from build123d import *

# Parameters (mm, degrees)
SKETCH1_R           = 52.5
BOSS_EXTRUDE1_DEPTH = 65


with BuildPart() as part:
    # Sketch1 → Boss-Extrude1 (new body)
    with BuildSketch(Plane(origin=(0, 0, 0), x_dir=(1, 0, 0), z_dir=(0, 1, 0))):
        with BuildLine():
            Line((0, 57), (0, 60))
            ThreePointArc((0, 60), (3.662912372, 59.888087905), (7.312160604, 59.552769098))
            Line((7.312160604, 59.552769098), (6.946552574, 56.575130644))
            ThreePointArc((6.946552574, 56.575130644), (9.407713534, 56.218279288), (11.850966377, 55.754413242))
            Line((11.850966377, 55.754413242), (12.474701449, 58.688856044))
            ThreePointArc((12.474701449, 58.688856044), (16.034302565, 57.817827193), (19.534089267, 56.731114536))
            Line((19.534089267, 56.731114536), (18.557384804, 53.894558809))
            ThreePointArc((18.557384804, 53.894558809), (20.890569923, 53.033801375), (23.183988655, 52.072091086))
            Line((23.183988655, 52.072091086), (24.404198585, 54.812727459))
            ThreePointArc((24.404198585, 54.812727459), (27.704916794, 53.220649991), (30.902284495, 51.430038042))
            Line((30.902284495, 51.430038042), (29.35717027, 48.85853614))
            ThreePointArc((29.35717027, 48.85853614), (31.460408163, 47.531491858), (33.503759381, 46.113968679))
            Line((33.503759381, 46.113968679), (35.267115138, 48.541019662))
            ThreePointArc((35.267115138, 48.541019662), (38.164693217, 46.297475003), (40.919901604, 43.881222097))
            Line((40.919901604, 43.881222097), (38.873906524, 41.687160992))
            ThreePointArc((38.873906524, 41.687160992), (40.655275602, 39.951828065), (42.359255052, 38.140444562))
            Line((42.359255052, 38.140444562), (44.588689529, 40.147836382))
            ThreePointArc((44.588689529, 40.147836382), (46.956489411, 37.350878198), (49.149122657, 34.414586181))
            Line((49.149122657, 34.414586181), (46.691666524, 32.693856872))
            ThreePointArc((46.691666524, 32.693856872), (48.073312411, 30.626077676), (49.363448016, 28.5))
            Line((49.363448016, 28.5), (51.961524227, 30))
            ThreePointArc((51.961524227, 30), (53.696061696, 26.771868787), (55.230291207, 23.443867709))
            Line((55.230291207, 23.443867709), (52.468776647, 22.271674324))
            ThreePointArc((52.468776647, 22.271674324), (53.390314787, 19.961820732), (54.210221429, 17.613968679))
            Line((54.210221429, 17.613968679), (57.063390978, 18.541019662))
            ThreePointArc((57.063390978, 18.541019662), (58.088858423, 15.022800243), (58.897631007, 11.448539723))
            Line((58.897631007, 11.448539723), (55.952749457, 10.876112736))
            ThreePointArc((55.952749457, 10.876112736), (56.373904212, 8.425136434), (56.687748036, 5.958122406))
            Line((56.687748036, 5.958122406), (59.671313722, 6.271707796))
            ThreePointArc((59.671313722, 6.271707796), (59.942893295, 2.617163242), (59.990861709, -1.047144386))
            Line((59.990861709, -1.047144386), (56.991318624, -0.994787167))
            ThreePointArc((56.991318624, -0.994787167), (56.89368351, -3.479766753), (56.687748036, -5.958122406))
            Line((56.687748036, -5.958122406), (59.671313722, -6.271707796))
            ThreePointArc((59.671313722, -6.271707796), (59.177136092, -9.902856352), (58.462203887, -13.497063261))
            Line((58.462203887, -13.497063261), (55.539093693, -12.822210098))
            ThreePointArc((55.539093693, -12.822210098), (54.926935833, -15.232587436), (54.210221429, -17.613968679))
            Line((54.210221429, -17.613968679), (57.063390978, -18.541019662))
            ThreePointArc((57.063390978, -18.541019662), (55.825054079, -21.990073603), (54.378467222, -25.357095704))
            Line((54.378467222, -25.357095704), (51.659543861, -24.089240919))
            ThreePointArc((51.659543861, -24.089240919), (50.559617491, -26.319670954), (49.363448016, -28.5))
            Line((49.363448016, -28.5), (51.961524227, -30))
            ThreePointArc((51.961524227, -30), (50.033149324, -33.116219119), (47.918130603, -36.108901389))
            Line((47.918130603, -36.108901389), (45.522224073, -34.30345632))
            ThreePointArc((45.522224073, -34.30345632), (43.982601253, -36.256458556), (42.359255052, -38.140444562))
            Line((42.359255052, -38.140444562), (44.588689529, -40.147836382))
            ThreePointArc((44.588689529, -40.147836382), (42.054555858, -42.795026949), (39.363541739, -45.282574813))
            Line((39.363541739, -45.282574813), (37.395364652, -43.018446073))
            ThreePointArc((37.395364652, -43.018446073), (35.483334288, -44.608664941), (33.503759381, -46.113968679))
            Line((33.503759381, -46.113968679), (35.267115138, -48.541019662))
            ThreePointArc((35.267115138, -48.541019662), (32.237976501, -50.603486749), (29.088577215, -52.477182428))
            Line((29.088577215, -52.477182428), (27.634148354, -49.853323307))
            ThreePointArc((27.634148354, -49.853323307), (25.433275347, -51.011258611), (23.183988655, -52.072091086))
            Line((23.183988655, -52.072091086), (24.404198585, -54.812727459))
            ThreePointArc((24.404198585, -54.812727459), (21.012442876, -56.200331355), (17.542302283, -57.378285358))
            Line((17.542302283, -57.378285358), (16.665187169, -54.50937109))
            ThreePointArc((16.665187169, -54.50937109), (14.271660231, -55.184415502), (11.850966377, -55.754413242))
            Line((11.850966377, -55.754413242), (12.474701449, -58.688856044))
            ThreePointArc((12.474701449, -58.688856044), (8.868564668, -59.340951802), (5.229344565, -59.771681886))
            Line((5.229344565, -59.771681886), (4.967877337, -56.783097791))
            ThreePointArc((4.967877337, -56.783097791), (2.48630508, -56.94574863), (0, -57))
            Line((0, -57), (0, -60))
            ThreePointArc((0, -60), (-3.662912372, -59.888087905), (-7.312160604, -59.552769098))
            Line((-7.312160604, -59.552769098), (-6.946552574, -56.575130644))
            ThreePointArc((-6.946552574, -56.575130644), (-9.407713534, -56.218279288), (-11.850966377, -55.754413242))
            Line((-11.850966377, -55.754413242), (-12.474701449, -58.688856044))
            ThreePointArc((-12.474701449, -58.688856044), (-16.034302565, -57.817827193), (-19.534089267, -56.731114536))
            Line((-19.534089267, -56.731114536), (-18.557384804, -53.894558809))
            ThreePointArc((-18.557384804, -53.894558809), (-20.890569923, -53.033801375), (-23.183988655, -52.072091086))
            Line((-23.183988655, -52.072091086), (-24.404198585, -54.812727459))
            ThreePointArc((-24.404198585, -54.812727459), (-27.704916794, -53.220649991), (-30.902284495, -51.430038042))
            Line((-30.902284495, -51.430038042), (-29.35717027, -48.85853614))
            ThreePointArc((-29.35717027, -48.85853614), (-31.460408163, -47.531491858), (-33.503759381, -46.113968679))
            Line((-33.503759381, -46.113968679), (-35.267115138, -48.541019662))
            ThreePointArc((-35.267115138, -48.541019662), (-38.164693217, -46.297475003), (-40.919901604, -43.881222097))
            Line((-40.919901604, -43.881222097), (-38.873906524, -41.687160992))
            ThreePointArc((-38.873906524, -41.687160992), (-40.655275602, -39.951828065), (-42.359255052, -38.140444562))
            Line((-42.359255052, -38.140444562), (-44.588689529, -40.147836382))
            ThreePointArc((-44.588689529, -40.147836382), (-46.956489411, -37.350878198), (-49.149122657, -34.414586181))
            Line((-49.149122657, -34.414586181), (-46.691666524, -32.693856872))
            ThreePointArc((-46.691666524, -32.693856872), (-48.073312411, -30.626077676), (-49.363448016, -28.5))
            Line((-49.363448016, -28.5), (-51.961524227, -30))
            ThreePointArc((-51.961524227, -30), (-53.696061696, -26.771868787), (-55.230291207, -23.443867709))
            Line((-55.230291207, -23.443867709), (-52.468776647, -22.271674324))
            ThreePointArc((-52.468776647, -22.271674324), (-53.390314787, -19.961820732), (-54.210221429, -17.613968679))
            Line((-54.210221429, -17.613968679), (-57.063390978, -18.541019662))
            ThreePointArc((-57.063390978, -18.541019662), (-58.088858423, -15.022800243), (-58.897631007, -11.448539723))
            Line((-58.897631007, -11.448539723), (-55.952749457, -10.876112736))
            ThreePointArc((-55.952749457, -10.876112736), (-56.373904212, -8.425136434), (-56.687748036, -5.958122406))
            Line((-56.687748036, -5.958122406), (-59.671313722, -6.271707796))
            ThreePointArc((-59.671313722, -6.271707796), (-59.942893295, -2.617163242), (-59.990861709, 1.047144386))
            Line((-59.990861709, 1.047144386), (-56.991318624, 0.994787167))
            ThreePointArc((-56.991318624, 0.994787167), (-56.89368351, 3.479766753), (-56.687748036, 5.958122406))
            Line((-56.687748036, 5.958122406), (-59.671313722, 6.271707796))
            ThreePointArc((-59.671313722, 6.271707796), (-59.177136092, 9.902856352), (-58.462203887, 13.497063261))
            Line((-58.462203887, 13.497063261), (-55.539093693, 12.822210098))
            ThreePointArc((-55.539093693, 12.822210098), (-54.926935833, 15.232587436), (-54.210221429, 17.613968679))
            Line((-54.210221429, 17.613968679), (-57.063390978, 18.541019662))
            ThreePointArc((-57.063390978, 18.541019662), (-55.825054079, 21.990073603), (-54.378467222, 25.357095704))
            Line((-54.378467222, 25.357095704), (-51.659543861, 24.089240919))
            ThreePointArc((-51.659543861, 24.089240919), (-50.559617491, 26.319670954), (-49.363448016, 28.5))
            Line((-49.363448016, 28.5), (-51.961524227, 30))
            ThreePointArc((-51.961524227, 30), (-50.033149324, 33.116219119), (-47.918130603, 36.108901389))
            Line((-47.918130603, 36.108901389), (-45.522224073, 34.30345632))
            ThreePointArc((-45.522224073, 34.30345632), (-43.982601253, 36.256458556), (-42.359255052, 38.140444562))
            Line((-42.359255052, 38.140444562), (-44.588689529, 40.147836382))
            ThreePointArc((-44.588689529, 40.147836382), (-42.054555858, 42.795026949), (-39.363541739, 45.282574813))
            Line((-39.363541739, 45.282574813), (-37.395364652, 43.018446073))
            ThreePointArc((-37.395364652, 43.018446073), (-35.483334288, 44.608664941), (-33.503759381, 46.113968679))
            Line((-33.503759381, 46.113968679), (-35.267115138, 48.541019662))
            ThreePointArc((-35.267115138, 48.541019662), (-32.237976501, 50.603486749), (-29.088577215, 52.477182428))
            Line((-29.088577215, 52.477182428), (-27.634148354, 49.853323307))
            ThreePointArc((-27.634148354, 49.853323307), (-25.433275347, 51.011258611), (-23.183988655, 52.072091086))
            Line((-23.183988655, 52.072091086), (-24.404198585, 54.812727459))
            ThreePointArc((-24.404198585, 54.812727459), (-21.012442876, 56.200331355), (-17.542302283, 57.378285358))
            Line((-17.542302283, 57.378285358), (-16.665187169, 54.50937109))
            ThreePointArc((-16.665187169, 54.50937109), (-14.271660231, 55.184415502), (-11.850966377, 55.754413242))
            Line((-11.850966377, 55.754413242), (-12.474701449, 58.688856044))
            ThreePointArc((-12.474701449, 58.688856044), (-8.868564668, 59.340951802), (-5.229344565, 59.771681886))
            Line((-5.229344565, 59.771681886), (-4.967877337, 56.783097791))
            ThreePointArc((-4.967877337, 56.783097791), (-2.48630508, 56.94574863), (0, 57))
        make_face()
        Circle(SKETCH1_R, mode=Mode.SUBTRACT)
    extrude(amount=BOSS_EXTRUDE1_DEPTH)


solid = part.part
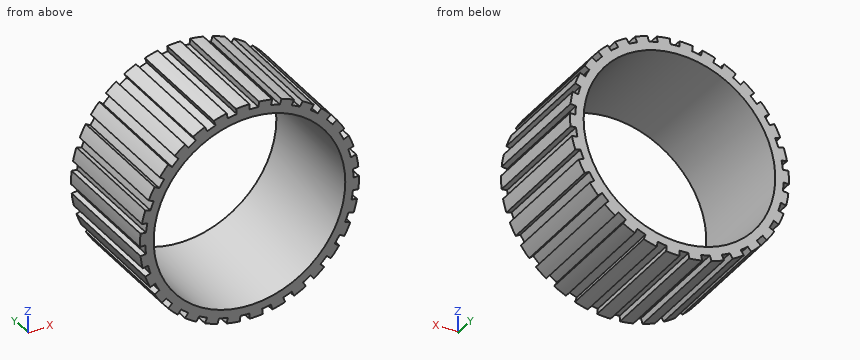
Build history of the part. All positions in model axes, mm. Round coordinates to 2 decimals unless told otherwise and drop trailing zeros. Loops run counter-clockwise (first coordinate to the right, second up) from the corner with the lowest first, then second, coordinate; pieces in that order, holes last. Notation, with made-up numbers: (36, -21) -> (67, -21) arc R10 cw to (67, -2) -> close; hole circle Ø4 at (-22.5, 47.5). An arc over 180 degrees is marked (long way). One line per item, written item: value. Start each with the question number.
Q1. Cut at B-B on x = 26. List the corners of the cut face in (y, z), plus the area to 3 significant figures.
Q2. Drop flat-ended pins along their axis: pin 1 Ø1 at (x, y) = (22, 32.5) entering from -Z; pin 2 Ø6 at (y, z) = (34.5, 26.5) entering from +X; pin 3 Ø8 at (x, y) = (19, 31.5) entering from -Z; pin 4 Ø4 at (x, z) = (39, -41.5) entering from -Y. Give the stop position or say it passes through.
Q3. Probe line 1 along X through (y, z) = (3, -47); line 2 along Z through (x, y) = (44.5, 16); line 3 along X through (y, z) = (38, 0). List the from-to ranges inside material, lowest first.
Q4. Cut at A-A on z = 8. List the corners of the cut face in (x, y).
Computed:
1. outline: (0, -54.07) -> (65, -54.07) -> (65, -45.61) -> (0, -45.61) -> close; (0, 45.61) -> (65, 45.61) -> (65, 50.72) -> (0, 50.72) -> close
1. area: 883 mm²
2. pin 1: z = -52.79
2. pin 2: x = 55.21
2. pin 3: z = -58.09
2. pin 4: y = 0
3. line 1: -34.15 to -23.39, 23.39 to 32.25, 34.15 to 37.3
3. line 2: -40.07 to -27.86, 27.86 to 35.62, 40.07 to 40.25
3. line 3: -60 to -52.5, 52.5 to 60
4. outline: (-56.44, 0) -> (-51.89, 0) -> (-51.89, 65) -> (-56.44, 65) -> close; (51.89, 0) -> (59.46, 0) -> (59.46, 65) -> (51.89, 65) -> close
